Verification items for the finished model (mm, model axes). A direction names the side the tool comes from. Give positions to 0.01 mm unless a question says otherwise; leave off trailing zeros. Order: outer loops, then holes, each group sorted by start corner. A loop starts at its lowest first (then second) coordinate and runs counter-clockwise, first axis right, second up. Notation, with made-up numbers: (31.25, 18) -> (45.25, 18) arc R15 cw to (45.25, 34) -> close; hole circle Ø4 at (76, -21). An arc over 180 degrees is marked (long way). Return JSON: item names as keys, results as strings. Group by question number.
(1) Depth check by flat-ended pin: pin 1 Ø4 at (x, y) = (62.52, 48.87) entering from +Z; pin 2 Ø5 at (y, z) = (47.5, 10.5) entering from +X; pin 3 Ø5 at (x, z) = (72, 8) entering from +Y. Enter the tip coordinate at first touch or a pass-through.
(2) Tool access check on faces 1 (the face through (74, 33, 13)), 2 (the face through (41, -106.628, 8)), 3 (the face through (49.018, -112, 8)), 4 (the face through (69.018, -77, 8)). Record the directions out of +Z, -Z, +X, -X, +Y, -Y that give a thin tool (end or side, any length) a straight path to the whole face; none if there is none.
(3) Cross-section at B-B on y = -78. Enter the section's corners in (x, z), then the cut area to 3 significant figures.
(4) Release check for a two-part mould opening along Y. For faces 5 (the face through (74, 41.372, 8)), 6 (the face through (-42.982, 48, 8)), 7 (the face through (74, 6.372, 8)) record: pulls with the +Y half, pulls with the -Y half, needs draft (parallel to the pull), parting line crosses it, or undercut.
(5) Cross-section at A-A on x = -38. Enter the section's corners in (y, z), then the cut area to 3 significant figures.
(6) Cross-section at D-D on x = 58.5. Enter the section's corners in (y, z).
(7) Cross-section at C-C on z = 6.75. State how many separate pieces and enclosed holes the cut face has, then the cut area to 3 significant figures.
(8) Thickness scan on line 1 along Y through (x, z) = (70.5, 3.5); line 2 along Y through (x, z) = (-22, 6.5); line 3 along X through (y, z) = (-108, 6). Record the ranges inside material, lowest first.
from build123d import *

# Parameters (mm, degrees)
SKETCH_1_W      = 128
SKETCH_1_H      = 170
SKETCH_1_R      = 1.5
EXTRUDE_1_DEPTH = 3
SKETCH_2_W      = 40
SKETCH_2_H      = 10
SKETCH_2_W_2    = 16
SKETCH_2_W_3    = 10
SKETCH_2_H_2    = 13
SKETCH_2_H_3    = 16
SKETCH_2_H_4    = 18
SKETCH_2_H_5    = 17
SKETCH_2_W_4    = 34
EXTRUDE_2_DEPTH = 10


with BuildPart() as part:
    # 草圖1 → 填料-伸長1 (new body)
    with BuildSketch(Plane.XY):
        with Locations((15.018050542, -31.628158845)):
            Rectangle(SKETCH_1_W, SKETCH_1_H)
        with Locations((-45.481949458, 48.871841155)):
            Circle(SKETCH_1_R, mode=Mode.SUBTRACT)
        with Locations((-45.481949458, -112.128158845)):
            Circle(SKETCH_1_R, mode=Mode.SUBTRACT)
        with Locations((73.018050542, -113.128158845)):
            Circle(SKETCH_1_R, mode=Mode.SUBTRACT)
        with Locations((62.518050542, 48.871841155)):
            Circle(SKETCH_1_R, mode=Mode.SUBTRACT)
    extrude(amount=EXTRUDE_1_DEPTH)

    # 草圖2 → 填料-伸長2 (add)
    with BuildSketch(Plane.XY.offset(3)):
        with Locations((-22.981949458, -111.628158845)):
            Rectangle(SKETCH_2_W, SKETCH_2_H)
        with Locations((41.018050542, -111.628158845)):
            Rectangle(SKETCH_2_W_2, SKETCH_2_H)
        with Locations((74.018050542, -90.128158845)):
            Rectangle(SKETCH_2_W_3, SKETCH_2_H_2)
        with Locations((74.018050542, -76.628158845)):
            Rectangle(SKETCH_2_W_3, SKETCH_2_H)
        with Locations((74.018050542, -38.628158845)):
            Rectangle(SKETCH_2_W_3, SKETCH_2_H_3)
        with Locations((74.018050542, -2.628158845)):
            Rectangle(SKETCH_2_W_3, SKETCH_2_H_4)
        with Locations((74.018050542, 32.871841155)):
            Rectangle(SKETCH_2_W_3, SKETCH_2_H_5)
        with Locations((31.018050542, 48.371841155)):
            Rectangle(SKETCH_2_W_4, SKETCH_2_H)
        with Locations((-22.981949458, 48.371841155)):
            Rectangle(SKETCH_2_W, SKETCH_2_H)
    extrude(amount=EXTRUDE_2_DEPTH)


solid = part.part
Verdict:
{
 "1": {"pin 1": "z = 3", "pin 2": "x = 48.02", "pin 3": "y = 41.37"},
 "2": {"face 1": "+Z, +X, -X, +Y, -Y", "face 2": "+Z, +X, -X", "face 3": "+Z, +X, +Y, -Y", "face 4": "+Z, -X, +Y, -Y"},
 "3": {"outline": "(-48.98, 0) -> (79.02, 0) -> (79.02, 13) -> (69.02, 13) -> (69.02, 3) -> (-48.98, 3) -> close", "area": "484 mm²"},
 "4": {"face 5": "pulls with the +Y half", "face 6": "needs draft", "face 7": "undercut"},
 "5": {"outline": "(-116.63, 0) -> (53.37, 0) -> (53.37, 13) -> (43.37, 13) -> (43.37, 3) -> (-106.63, 3) -> (-106.63, 13) -> (-116.63, 13) -> close", "area": "710 mm²"},
 "6": {"outline": "(-116.63, 0) -> (53.37, 0) -> (53.37, 3) -> (-116.63, 3) -> close"},
 "7": {"separate pieces": "9", "enclosed holes": "0", "area": "2,040 mm²"},
 "8": {"line 1": "-96.63 to -83.63, -81.63 to -71.63, -46.63 to -30.63, -11.63 to 6.37, 24.37 to 41.37", "line 2": "-116.63 to -106.63, 43.37 to 53.37", "line 3": "-42.98 to -2.98, 33.02 to 49.02"}
}
